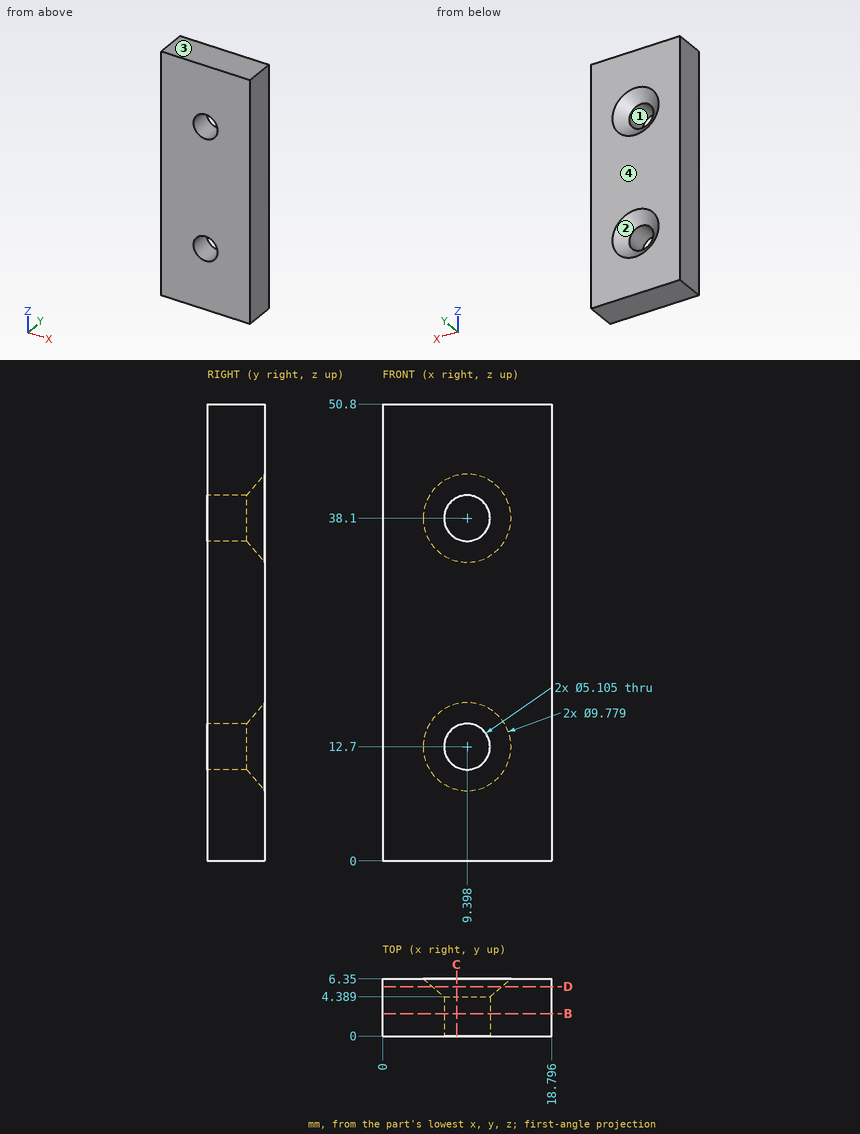
Design review of the part shown in the three views and the two pictorial views. Dimensions are in mm from the part's minimum x, y and z. Round coordinates to 2 decimals unless told otherwise and drop trailing zeros. Order: outer loops, then holes, each group sorted by start corner. A loop starts at its lowest first (then second) coordinate and runs counter-clockwise, first axis right, second up. Notation, with made-up numbers: (-39, -22.5) -> (1, -22.5) arc R25 cw to (1, 11.5) -> close; hole circle Ø6 at (88, 1.5). An arc over 180 degrees is marked (long way). Write item = value, one per line. Start each with the question number.
1) Take a section at B-B on y = 2.5. State the section outline as (x, z) points (1 decimal), plus the area to 3 significant figures.
2) To check wall thickness, follow line 1 (Z direction, x = 9.5, y = 4.5) (1 decimal); line 2 (Z direction, x = 7.25, y = 2.75); line 3 (Y direction, x = 9.5, z = 10) (1 decimal). State the ranges of each line that lie inside material, in increasing order. Write a range as from..to.
3) The part is to be moulded in two halves that separate along Z. For the marked faces 1, 2, 3 and 4, say which applies: +Z half, -Z half, draft (parallel to the pull), parting line (faces both ways), or undercut.
4) Insertion check: pin 1 (6.5 mm diameter, centred on x = 9.398, z = 38.1, fed in from +Y) (1 decimal). The pin has a flat end and moves straight along its axis. Give the tip position at first contact, or say it passes through.
5) Take a section at C-C on x = 8.25. Count the separate pieces of the cut face and the enclosed holes in it, plus the area to 3 significant figures.
6) Take a section at D-D on y = 5.5. State the section outline as (x, z) points.
Verdict:
q1.outline = (0, 0) -> (18.8, 0) -> (18.8, 50.8) -> (0, 50.8) -> close; hole circle Ø5.1 at (9.4, 12.7); hole circle Ø5.1 at (9.4, 38.1)
q1.area = 914 mm2
q2.line_1 = 0..10, 15.4..35.4, 40.8..50.8
q2.line_2 = 0..11.32, 14.08..36.72, 39.48..50.8
q2.line_3 = 0..4.5
q3.face_1 = undercut
q3.face_2 = undercut
q3.face_3 = +Z half
q3.face_4 = draft
q4.pin_1 = 5
q5.separate_pieces = 3
q5.enclosed_holes = 0
q5.area = 255 mm2
q6.outline = (0, 0) -> (18.8, 0) -> (18.8, 50.8) -> (0, 50.8) -> close; hole circle Ø7.75 at (9.4, 12.7); hole circle Ø7.75 at (9.4, 38.1)
